```python
from build123d import *

# Parameters (mm, degrees)
SKETCH1_W           = 300
SKETCH1_H           = 200
SKETCH1_R           = 20
BOSS_EXTRUDE2_DEPTH = 5
FILLET1_R           = 10


with BuildPart() as part:
    # Sketch1 → Boss-Extrude2 (new body)
    with BuildSketch(Plane(origin=(0, 0, 0), x_dir=(1, 0, 0), z_dir=(0, 1, 0))):
        Rectangle(SKETCH1_W, SKETCH1_H)
        with Locations(Location((-45, 0, 0), (0, 0, 270))):
            Circle(SKETCH1_R, mode=Mode.SUBTRACT)
        Polygon((-88.055456352, 80.126524164), (-95.126524164, 73.055456352), (-91.944543648, 69.873475836), (-84.873475836, 76.944543648), align=None, mode=Mode.SUBTRACT)
        Polygon((-121.944543648, 39.873475836), (-114.873475836, 46.944543648), (-118.055456352, 50.126524164), (-125.126524164, 43.055456352), align=None, mode=Mode.SUBTRACT)
        Polygon((-1.944543648, 80.126524164), (5.126524164, 73.055456352), (1.944543648, 69.873475836), (-5.126524164, 76.944543648), align=None, mode=Mode.SUBTRACT)
        Polygon((35.126524164, 43.055456352), (28.055456352, 50.126524164), (24.873475836, 46.944543648), (31.944543648, 39.873475836), align=None, mode=Mode.SUBTRACT)
        Polygon((-1.944543648, -80.126524164), (5.126524164, -73.055456352), (1.944543648, -69.873475836), (-5.126524164, -76.944543648), align=None, mode=Mode.SUBTRACT)
        Polygon((35.126524164, -43.055456352), (28.055456352, -50.126524164), (24.873475836, -46.944543648), (31.944543648, -39.873475836), align=None, mode=Mode.SUBTRACT)
        Polygon((-125.126524164, -43.055456352), (-118.055456352, -50.126524164), (-114.873475836, -46.944543648), (-121.944543648, -39.873475836), align=None, mode=Mode.SUBTRACT)
        Polygon((-88.055456352, -80.126524164), (-95.126524164, -73.055456352), (-91.944543648, -69.873475836), (-84.873475836, -76.944543648), align=None, mode=Mode.SUBTRACT)
        Polygon((15.176776695, 56.641242789), (11.641242789, 60.176776695), (14.823223305, 63.358757211), (18.358757211, 59.823223305), align=None, mode=Mode.SUBTRACT)
        Polygon((15.176776695, -56.641242789), (11.641242789, -60.176776695), (14.823223305, -63.358757211), (18.358757211, -59.823223305), align=None, mode=Mode.SUBTRACT)
        Polygon((-101.641242789, -60.176776695), (-105.176776695, -56.641242789), (-108.358757211, -59.823223305), (-104.823223305, -63.358757211), align=None, mode=Mode.SUBTRACT)
        Polygon((-105.176776695, 56.641242789), (-101.641242789, 60.176776695), (-104.823223305, 63.358757211), (-108.358757211, 59.823223305), align=None, mode=Mode.SUBTRACT)
    extrude(amount=BOSS_EXTRUDE2_DEPTH)

    # Fillet1
    fillet1_edges = [part.edges().sort_by_distance(p)[0] for p in [
        (-150, 2.5, -100),
        (150, 2.5, -100),
        (150, 2.5, 100),
        (-150, 2.5, 100),
    ]]
    fillet(fillet1_edges, radius=FILLET1_R)


solid = part.part
```
Check sheet for the modelled part. Datum: model origin and axes. Units: mm. A direction names the side the tool comes from. Round coordinates to 2 decimals unless told otherwise and drop trailing zeros. Order: outer loops, then holes, each group sorted by start corner. A loop starts at its lowest first (then second) coordinate and runs counter-clockwise, first axis right, second up. Notation, with made-up numbers: (-39.75, 44.5) -> (-20.75, 44.5) arc R20 ccw to (-20.75, 69.5) -> close; hole circle Ø9 at (32.25, 60). An arc over 180 degrees is marked (long way). One line per item, written item: value. Start each with the question number.
Q1. Gauge pin test, flat ends, axial feed: pin 1 Ø1 at (x, z) = (8.5, -37) entering from -Y; pin 2 Ø24 at (x, z) = (-45, 0) entering from -Y. Record the tip position at first contact, or that the pin passes through.
Q2. Set-up check for faces 1 (the face through (146.99, 2.54, 97.15)), 2 (the face through (1.54, 2.46, -76.64)): record each of +Z, -Z, +X, -X, +Y, -Y from which the full face is reachable in a straight line by a thin tool's end or side.
Q3. Cross-section at A-A (z = 0). Record the boundary of the cut face in (x, y).
Q4. Cross-section at B-B (x = -45). Record the boundary of the cut face in (y, z).
Q5. Cross-section at C-C (y = 1.5). Give the number of separate pieces and of enclosed holes in the cut face, and give its area (3 significant figures).
Q6. Thickness scan on line 1 (X direction, y = 2.25, z = 0); line 2 (Z direction, x = -90.5, y = 3.5); line 3 (X direction, y = 3.1, z = -72). Record the ranges inside material, lowest first.
Completed:
1. pin 1: stops at y = 0
1. pin 2: passes through
2. face 1: +Z, +X, +Y, -Y
2. face 2: +Y, -Y
3. outline: (-150, 0) -> (-65, 0) -> (-65, 5) -> (-150, 5) -> close; (-25, 0) -> (150, 0) -> (150, 5) -> (-25, 5) -> close
4. outline: (0, -100) -> (5, -100) -> (5, -20) -> (0, -20) -> close; (0, 20) -> (5, 20) -> (5, 100) -> (0, 100) -> close
5. separate pieces: 1
5. enclosed holes: 13
5. area: 58,200 mm²
6. line 1: x = -150 to -65, -25 to 150
6. line 2: z = -100 to -77.68, -71.32 to 71.32, 77.68 to 100
6. line 3: x = -150 to -94.07, -89.82 to -0.18, 4.07 to 150
